Verification items for this drawing (mm, ordinates from the low corner). A direction names the side the tool comes from. Coordinates: 2 decimals unless noted, no trailing zeros. Order: outer loops, then holes, each group sorted by start corner. A loop starts at its lowest first (then second) coordinate and runs counter-clockwise, first axis right, second up. Notation, with made-up numbers: M -25.5,-0.75 L 14.5,-0.75 A24 ccw 14.5,19.25 Z; hole C 32,41.25 d8. An arc over 180 degrees is marked long. Use CSV: the item, a comma, the result in double quotes. Start each with the question number.
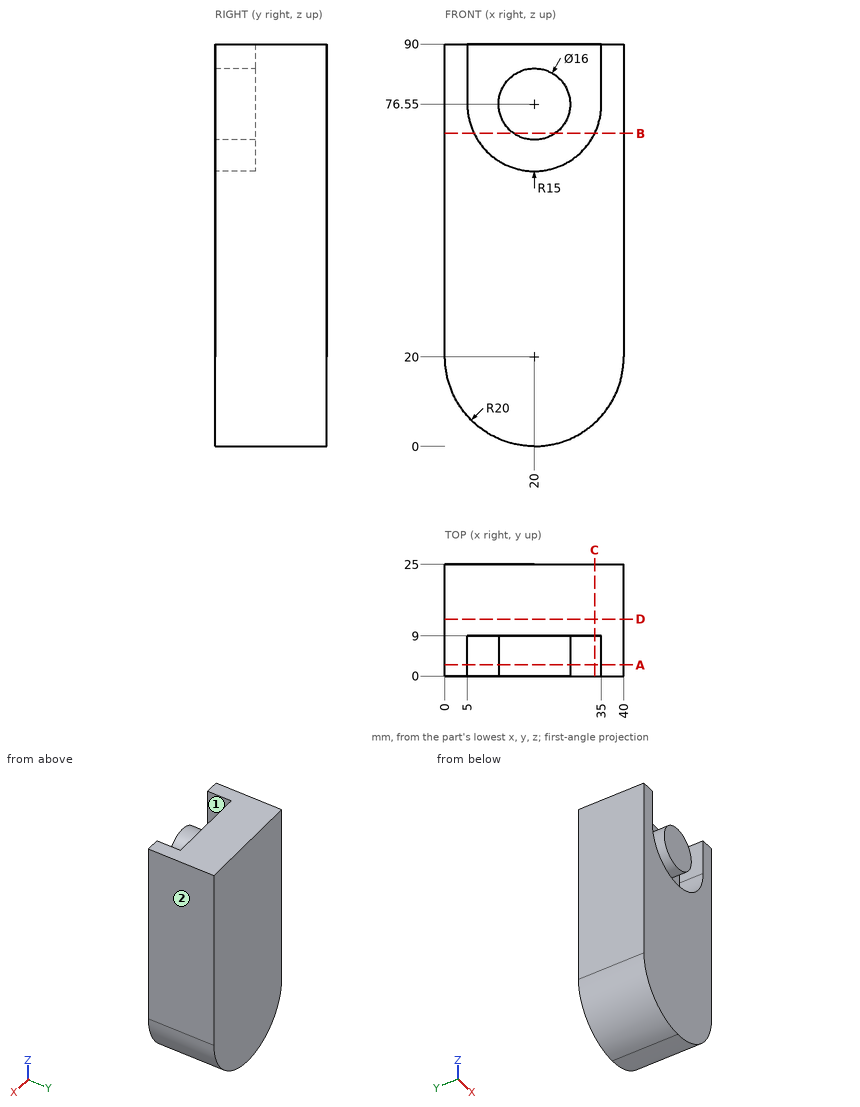
1) Section check C-C on x = 33.5. Record the boundary of the cut face in (y, z).
2) Section check B-B on z = 70. Record the boundary of the cut face in (x, y) (1 decimal), then the cut area to 3 significant figures.
3) Material ranges on line 1 along Y through (x, z) = (13, 82); line 2 along X through (y, z) = (2.5, 73) (1 decimal); line 3 along Z through (x, y) = (26, 6.75), recorded low to high.
4) Section check D-D on y = 12.75. Record the boundary of the cut face in (x, z), then the cut area to 3 significant figures.
5) Section check A-A on y = 2.5. Record the boundary of the cut face in (x, z), then the cut area to 3 significant figures.
6) Gauge pin test, flat ends, axial feed: P1, Ø1.5, axis at x = 21, y = 17, coming from the -Z side; P2, Ø4, axis at y = 13, z = 9.5, coming from the +X side. Record the tip position at first contact, or that the pin passes through.
7) Set-up check for the marked faces 1 and 2: record each of +Z, -Z, +X, -X, +Y, -Y from which the full face is reachable in a straight line by a thin tool's end or side.
Results are:
1,outline,"M 0,5.24 L 25,5.24 L 25,90 L 9,90 L 9,70.01 L 0,70.01 Z"
2,outline,"M 0,0 L 6.5,0 L 6.5,9 L 15.4,9 L 15.4,0 L 24.6,0 L 24.6,9 L 33.5,9 L 33.5,0 L 40,0 L 40,25 L 0,25 Z"
2,area,"840 mm²"
3,line 1,"y = 9 to 25"
3,line 2,"x = 0 to 5.4, 12.8 to 27.2, 34.6 to 40"
3,line 3,"z = 0.92 to 62.8, 71.26 to 81.84"
4,outline,"M 0,20 A20 ccw 40,20 L 40,90 L 0,90 Z"
4,area,"3,430 mm²"
5,outline,"M 0,20 A20 ccw 40,20 L 40,90 L 35,90 L 35,76.55 A15 cw 5,76.55 L 5,90 L 0,90 Z; C 20,76.55 d16"
5,area,"2,870 mm²"
6,P1,"stops at z = 0"
6,P2,"stops at x = 38.1"
7,face 1,"+Z, -Y"
7,face 2,"+Z, -Z, +X, +Y, -Y"
